```python
from build123d import *

# Parameters (mm, degrees)
F0_W            = 20
F0_H            = 20
F0_R            = 1.8
F1_DEPTH        = 11
F2_W            = 13
F2_H            = 2.5
F2_W_2          = 2.5
F2_H_2          = 13
F3_DEPTH        = 14
F2_R            = 2.5
F2_R_2          = 1.8
F4_DEPTH        = 1
F5_W            = 2.5
F5_H            = 6.5
F6_DEPTH        = 25
F8_DEPTH        = 13
F8_COPIES_COUNT = 4


# Not quite as in the source:
# - a pattern or mirror of a feature is missing from the dataset's text; its kind, count and spacing are read off the source's solid


with BuildPart() as f1:
    # F0 (on Right) → F1 (new body)
    with BuildSketch(Plane.YZ):
        Rectangle(F0_W, F0_H)
        Circle(F0_R, mode=Mode.SUBTRACT)
    extrude(amount=-F1_DEPTH)

    # F2 (on face) → F3 (join)
    with BuildSketch(Plane(origin=(-11, 0, 0), x_dir=(0, -1, 0), z_dir=(-1, 0, 0))):
        with Locations((0, -8.75)):
            Rectangle(F2_W, F2_H)
        with Locations((8.75, 0)):
            Rectangle(F2_W_2, F2_H_2)
        with Locations((-8.75, 0)):
            Rectangle(F2_W_2, F2_H_2)
        with Locations((0, 8.75)):
            Rectangle(F2_W, F2_H)
    extrude(amount=F3_DEPTH)

    # F2 (on face) → F4 (cut)
    with BuildSketch(Plane(origin=(-11, 0, 0), x_dir=(0, -1, 0), z_dir=(-1, 0, 0))):
        Circle(F2_R)
        Circle(F2_R_2, mode=Mode.SUBTRACT)
    extrude(amount=-F4_DEPTH, mode=Mode.SUBTRACT)

    # F5 (on face) → F6 (cut)
    with BuildSketch(Plane.XZ.offset(10)):
        with Locations((-7.75, 0)):
            Rectangle(F5_W, F5_H)
    extrude(amount=-F6_DEPTH, mode=Mode.SUBTRACT)

    # F7 (on face) → F8 (join, through all)
    with BuildSketch(Plane.XZ.offset(6.5)):
        with BuildLine():
            Line((-25, -7.5), (-22.3846606339, -7.5))
            ThreePointArc((-22.3846606339, -7.5), (-23.6923303169, -7.2), (-25, -7.5))
        make_face()
    f8 = extrude(amount=-F8_DEPTH)

    # F8_copies: F8 ×4 about axis
    f8_copies_axis = Axis((0, 0, 0), (1, 0, 0))
    for i in range(1, F8_COPIES_COUNT):
        add(f8.rotate(f8_copies_axis, i * 360 / F8_COPIES_COUNT))


solid = f1.part
```
Source: CAD feature listing. Evaluate the final solid. Frame: model axes, mm. A direction names the side the tool comes from. Give positions to 0.01 mm unless a question says otherwise; leave off trailing zeros. Loops run counter-clockwise (first coordinate to the right, second up) from the corner with the lowest first, then second, coordinate; pieces in that order, holes last. Notation, with made-up numbers: (-28, 28.5) -> (-2, 28.5) arc R32 cw to (-2, 55.5) -> close; hole circle Ø5 at (80.25, 70). An arc over 180 degrees is marked (long way). Use a Markdown table: item, result. Add a question column.
(1) Access query for faces 5 (the face through (-18, -9, -6.5)), 6 (the face through (-8, 0, 3.25)), 7 (the face through (-18, -9, 6.5)), 8 (the face through (-17, 7.5, 0)), 9 (the face through (-10.51, 0.54, -2.44)). Directions: +Z, -Z, +X, -X, +Y, -Y. A direction counts if a zero-diameter tool reaches every point of the face in a straight line with its end or side. Return the directions, or none.
(2) Section query A-A (x = -14). Output: boundary loops of the cut face in (y, z).
(3) Section query D-D (z = 6). Output: boundary loops of the cut face in (x, y).
(4) Ray query, line 1 (Z direction, x = -7, y = 9); line 2 (Z direction, x = -10.25, y = 0); line 3 (X direction, y = 1.75, z = -1.75). Return the intervals inside material, ascending.
(5) Section query B-B (y = 0). Output: boundary loops of the cut face in (x, z).
(6) Pull-direction query (X, two-part tool) for faces 1 (the face through (-23.7, -7.2, 0.1)), 2 (the face through (-10, 1, 2)), 3 (the face through (-18, 6.5, 9)), 4 (the face through (-17, 0, 7.5)); classes: +X half, -X half, draft (parallel to the pull), parting line (faces both ways), or undercut.
(7) First-contact query: pin 1 Ø0.8 at (x, y) = (-15, -8) entering from +Z; pin 2 Ø3 at (x, z) = (-17, -9) entering from +Y; pin 3 Ø1.4 at (x, z) = (-15.5, 9) entering from -Y; pin 4 Ø3 at (y, z) = (0, 0) entering from +X. Flat tips, straight axial feed; report the tip coordinate or a pass-through.
(8) Section query C-C (z = 0). Output: boundary loops of the cut face in (x, y).
Checked values:
| question | item | result |
|---|---|---|
| 1 | face 5 | -Z, -X, +Y, -Y |
| 1 | face 6 | +Y, -Y |
| 1 | face 7 | +Z, -X, +Y, -Y |
| 1 | face 8 | +Z, -Z |
| 1 | face 9 | -X |
| 2 | outline | (-10, -6.5) -> (-7.5, -6.5) -> (-7.5, 6.5) -> (-10, 6.5) -> close; (-6.5, -10) -> (6.5, -10) -> (6.5, -7.5) -> (-6.5, -7.5) -> close; (-6.5, 7.5) -> (6.5, 7.5) -> (6.5, 10) -> (-6.5, 10) -> close; (7.5, -6.5) -> (10, -6.5) -> (10, 6.5) -> (7.5, 6.5) -> close |
| 3 | outline | (-25, -10) -> (0, -10) -> (0, 10) -> (-25, 10) -> (-25, 7.5) arc R3 ccw to (-22.38, 7.5) -> (-11, 7.5) -> (-11, -7.5) -> (-22.38, -7.5) arc R3 ccw to (-25, -7.5) -> close |
| 4 | line 1 | -10 to -3.25, 3.25 to 10 |
| 4 | line 2 | -10 to -2.5, 2.5 to 10 |
| 4 | line 3 | -10 to -9, -6.5 to 0 |
| 5 | outline | (-25, -10) -> (0, -10) -> (0, -1.8) -> (-6.5, -1.8) -> (-6.5, -3.25) -> (-9, -3.25) -> (-9, -1.8) -> (-10, -1.8) -> (-10, -2.5) -> (-11, -2.5) -> (-11, -7.5) -> (-22.38, -7.5) arc R3 ccw to (-25, -7.5) -> close; (-25, 7.5) arc R3 ccw to (-22.38, 7.5) -> (-11, 7.5) -> (-11, 2.5) -> (-10, 2.5) -> (-10, 1.8) -> (-9, 1.8) -> (-9, 3.25) -> (-6.5, 3.25) -> (-6.5, 1.8) -> (0, 1.8) -> (0, 10) -> (-25, 10) -> close |
| 6 | face 1 | undercut |
| 6 | face 2 | -X half |
| 6 | face 3 | draft |
| 6 | face 4 | undercut |
| 7 | pin 1 | z = 6.5 |
| 7 | pin 2 | y = 6.5 |
| 7 | pin 3 | y = -6.5 |
| 7 | pin 4 | through |
| 8 | outline | (-25, -10) -> (-9, -10) -> (-9, -1.8) -> (-10, -1.8) -> (-10, -2.5) -> (-11, -2.5) -> (-11, -7.5) -> (-22.38, -7.5) arc R3 ccw to (-25, -7.5) -> close; (-25, 7.5) arc R3 ccw to (-22.38, 7.5) -> (-11, 7.5) -> (-11, 2.5) -> (-10, 2.5) -> (-10, 1.8) -> (-9, 1.8) -> (-9, 10) -> (-25, 10) -> close; (-6.5, -10) -> (0, -10) -> (0, -1.8) -> (-6.5, -1.8) -> close; (-6.5, 1.8) -> (0, 1.8) -> (0, 10) -> (-6.5, 10) -> close |
